CAD build for the part. Positions are in the model's coordinates, mm. A direction names the side the tool comes from. Coordinates: 2 decimals unless noted, no trailing zeros. Loops run counter-clockwise (first coordinate to the right, second up) from the corner with the lowest first, then second, coordinate; pieces in that order, holes last. Notation, with made-up numbers: (17.25, -17.5) -> (37.25, -17.5) arc R25 cw to (37.25, 21.5) -> close; hole circle Ø5 at (-27, 44). An arc over 180 degrees is marked (long way). Return JSON: item names as keys, results as strings. Group by question number.
(1) Probe L1, parallel to Z at x = 0, y = -8; L2, parallel to Y at x = -3.5, z = 11; L3, parallel to X at y = -13.75, z = 10. List the from-to ranges inside material, lowest first.
(2) Mould opens along X. For faces 1 (the face through (15.273, -7.395, -7.126)), 2 (the face through (-15.349, -7.395, -7.108)), 3 (the face through (2.69, -14.88, -5.18)) say: pulls with the +X half, pulls with the -X half, needs draft (parallel to the pull), parting line crosses it, or undercut.
(3) Tool access for faces 4 (the face through (-3, -13, 0)), 5 (the face through (2.057, -7.395, 16.727)), 6 (the face through (-12.34, -7.4, -8.94)), 7 (the face through (-4.731, -7.395, -14.487)): list every direction of +Z, -Z, +X, -X, +Y, -Y with a clear straight run to the whole face (end or side of a thin tool).
(4) Flat gauge pins, fed straight in: pin 1 Ø2 at (x, z) = (-5, 14.5) entering from +Y; pin 2 Ø1 at (x, y) = (-10, -3) entering from +Z; pin 3 Ø4 at (y, z) = (-7, 1.5) entering from -X; pin 4 Ø2 at (x, z) = (-3, -9.5) entering from -Y. Where does each tip first touch, or does it go through?
(5) Saw through at A-A on x = 12.5. Write the cut outline in (y, z).
```python
from build123d import *

# Parameters (mm, degrees)
F1_DEPTH = 15
F2_SIZE  = 0.5
F3_SIZE  = 4
F4_R     = 2
F5_DEPTH = 25.4
F6_R     = 3
F7_DEPTH = 5
F8_R     = 14.605
F8_R_2   = 3.175
F9_DEPTH = 2.54


# Not quite as in the source:
# - a fillet or chamfer that OpenCascade refuses, or shapes differently, is made with other operations: its cross-section is extruded or revolved along the edge and cut away or added


with BuildPart() as f1:
    # F0 (on Front) → F1 (new body)
    with BuildSketch(Plane.XZ):
        with BuildLine():
            Line((0, -20.1), (3.1676147888, -14.9071733253))
            ThreePointArc((3.1676147888, -14.9071733253), (0, -15.24), (-3.1676147888, -14.9071733253))
            Line((-3.1676147888, -14.9071733253), (0, -20.1))
        make_face()
        with BuildLine():
            ThreePointArc((-3.1676147888, 14.9071733253), (0, 15.24), (3.1676147888, 14.9071733253))
            Line((3.1676147888, 14.9071733253), (0, 20.1))
            Line((0, 20.1), (-3.1676147888, 14.9071733253))
        make_face()
        with BuildLine():
            ThreePointArc((-11.3248708297, 10.1982793004), (-8.9578472449, 12.3294189943), (-6.1995624382, 13.922033816))
            Line((-6.1995624382, 13.922033816), (-11.8144835711, 16.2612415869))
            Line((-11.8144835711, 16.2612415869), (-11.3248708297, 10.1982793004))
        make_face()
        with BuildLine():
            ThreePointArc((-15.1564111319, 1.5939892096), (-14.4941013083, 4.7094189943), (-13.1987175292, 7.6191505816))
            Line((-13.1987175292, 7.6191505816), (-19.1162359775, 6.2112415869))
            Line((-19.1162359775, 6.2112415869), (-15.1564111319, 1.5939892096))
        make_face()
        with BuildLine():
            Line((-19.1162359775, -6.2112415869), (-13.1987175292, -7.6191505816))
            ThreePointArc((-13.1987175292, -7.6191505816), (-14.4941013083, -4.7094189943), (-15.1564111319, -1.5939892096))
            Line((-15.1564111319, -1.5939892096), (-19.1162359775, -6.2112415869))
        make_face()
        with BuildLine():
            Line((-11.8144835711, -16.2612415869), (-6.1995624382, -13.922033816))
            ThreePointArc((-6.1995624382, -13.922033816), (-8.9578472449, -12.3294189943), (-11.3248708297, -10.1982793004))
            Line((-11.3248708297, -10.1982793004), (-11.8144835711, -16.2612415869))
        make_face()
        with BuildLine():
            ThreePointArc((15.1564111319, -1.5939892096), (15.2190884361, -0.7980897035), (15.24, 0))
            ThreePointArc((15.24, 0), (15.2190884361, 0.7980897035), (15.1564111319, 1.5939892096))
            ThreePointArc((15.1564111319, 1.5939892096), (14.4941013083, 4.7094189943), (13.1987175292, 7.6191505816))
            ThreePointArc((13.1987175292, 7.6191505816), (12.3294189943, 8.9578472449), (11.3248708297, 10.1982793004))
            ThreePointArc((11.3248708297, 10.1982793004), (8.9578472449, 12.3294189943), (6.1995624382, 13.922033816))
            ThreePointArc((6.1995624382, 13.922033816), (4.7094189943, 14.4941013083), (3.1676147888, 14.9071733253))
            ThreePointArc((3.1676147888, 14.9071733253), (0, 15.24), (-3.1676147888, 14.9071733253))
            ThreePointArc((-3.1676147888, 14.9071733253), (-4.7094189943, 14.4941013083), (-6.1995624382, 13.922033816))
            ThreePointArc((-6.1995624382, 13.922033816), (-8.9578472449, 12.3294189943), (-11.3248708297, 10.1982793004))
            ThreePointArc((-11.3248708297, 10.1982793004), (-12.3294189943, 8.9578472449), (-13.1987175292, 7.6191505816))
            ThreePointArc((-13.1987175292, 7.6191505816), (-14.4941013083, 4.7094189943), (-15.1564111319, 1.5939892096))
            ThreePointArc((-15.1564111319, 1.5939892096), (-15.24, 0), (-15.1564111319, -1.5939892096))
            ThreePointArc((-15.1564111319, -1.5939892096), (-14.4941013083, -4.7094189943), (-13.1987175292, -7.6191505816))
            ThreePointArc((-13.1987175292, -7.6191505816), (-12.3294189943, -8.9578472449), (-11.3248708297, -10.1982793004))
            ThreePointArc((-11.3248708297, -10.1982793004), (-8.9578472449, -12.3294189943), (-6.1995624382, -13.922033816))
            ThreePointArc((-6.1995624382, -13.922033816), (-4.7094189943, -14.4941013083), (-3.1676147888, -14.9071733253))
            ThreePointArc((-3.1676147888, -14.9071733253), (0, -15.24), (3.1676147888, -14.9071733253))
            ThreePointArc((3.1676147888, -14.9071733253), (4.7094189943, -14.4941013083), (6.1995624382, -13.922033816))
            ThreePointArc((6.1995624382, -13.922033816), (8.9578472449, -12.3294189943), (11.3248708297, -10.1982793004))
            ThreePointArc((11.3248708297, -10.1982793004), (12.3294189943, -8.9578472449), (13.1987175292, -7.6191505816))
            ThreePointArc((13.1987175292, -7.6191505816), (14.4941013083, -4.7094189943), (15.1564111319, -1.5939892096))
        make_face()
        with BuildLine():
            ThreePointArc((6.1995624382, 13.922033816), (8.9578472449, 12.3294189943), (11.3248708297, 10.1982793004))
            Line((11.3248708297, 10.1982793004), (11.8144835711, 16.2612415869))
            Line((11.8144835711, 16.2612415869), (6.1995624382, 13.922033816))
        make_face()
        with BuildLine():
            ThreePointArc((13.1987175292, 7.6191505816), (14.4941013083, 4.7094189943), (15.1564111319, 1.5939892096))
            Line((15.1564111319, 1.5939892096), (19.1162359775, 6.2112415869))
            Line((19.1162359775, 6.2112415869), (13.1987175292, 7.6191505816))
        make_face()
        with BuildLine():
            Line((19.1162359775, -6.2112415869), (15.1564111319, -1.5939892096))
            ThreePointArc((15.1564111319, -1.5939892096), (14.4941013083, -4.7094189943), (13.1987175292, -7.6191505816))
            Line((13.1987175292, -7.6191505816), (19.1162359775, -6.2112415869))
        make_face()
        with BuildLine():
            Line((11.8144835711, -16.2612415869), (11.3248708297, -10.1982793004))
            ThreePointArc((11.3248708297, -10.1982793004), (8.9578472449, -12.3294189943), (6.1995624382, -13.922033816))
            Line((6.1995624382, -13.922033816), (11.8144835711, -16.2612415869))
        make_face()
    extrude(amount=F1_DEPTH)

    # F2
    f2_edges = [f1.edges().sort_by_distance(p)[0] for p in [
        (0, -7.5, -20.1),
        (0, -7.5, 20.1),
        (-11.814484, -7.5, -16.261242),
        (-19.116236, -7.5, -6.211242),
        (-19.116236, -7.5, 6.211242),
        (-11.814484, -7.5, 16.261242),
        (11.814484, -7.5, 16.261242),
        (19.116236, -7.5, 6.211242),
        (19.116236, -7.5, -6.211242),
        (11.814484, -7.5, -16.261242),
    ]]
    chamfer(f2_edges, length=F2_SIZE)

    # F3
    f3_edges = [f1.edges().sort_by_distance(p)[0] for p in [
        (-11.563586, -15, 15.915911),
        (-11.563586, 0, 15.915911),
        (0, 0, 19.673148),
        (0, -15, 19.673148),
        (0, -15, -19.673148),
        (-11.563586, -15, -15.915911),
        (-18.710275, -15, -6.079337),
        (-18.710275, -15, 6.079337),
        (-18.710275, 0, 6.079337),
        (-18.710275, 0, -6.079337),
        (-11.563586, 0, -15.915911),
        (0, 0, -19.673148),
        (11.563586, -15, 15.915911),
        (18.710275, -15, 6.079337),
        (18.710275, -15, -6.079337),
        (11.563586, -15, -15.915911),
        (11.563586, 0, 15.915911),
        (18.710275, 0, 6.079337),
        (18.710275, 0, -6.079337),
        (11.563586, 0, -15.915911),
    ]]
    chamfer(f3_edges, length=F3_SIZE)

    # F4 (on face) → F5 (cut)
    with BuildSketch(Plane.XZ.offset(15)):
        Circle(F4_R)
    extrude(amount=-F5_DEPTH, mode=Mode.SUBTRACT)

    # F6 (on face) → F7 (cut)
    with BuildSketch(Plane.XZ.offset(15)):
        Circle(F6_R)
    extrude(amount=-F7_DEPTH, mode=Mode.SUBTRACT)

    # F8 (on face) → F9 (cut)
    with BuildSketch(Plane.XZ.offset(15)):
        Circle(F8_R)
        Circle(F8_R_2, mode=Mode.SUBTRACT)
    extrude(amount=-F9_DEPTH, mode=Mode.SUBTRACT)

    # F10: chamfer of 5.08 on 1 edges, made by hand


with BuildPart() as f10_tool2:
    # F10_s3 → F10_t4 (revolve)
    with BuildSketch(Plane.XY):
        Polygon((8.255, -12.46), (3.175, -17.54), (3.175, -12.46), align=None)
    revolve(axis=Axis((0, -12.46, 0), (0, -1, 0)))

    split(bisect_by=Plane.XZ.offset(15), keep=Keep.BOTTOM)


with BuildPart() as f1_1:
    add(f1.part)

    # F10_t1: union F10_tool2
    add(f10_tool2.part)


solid = f1_1.part
```
Geometry results:
{
 "1": {"L1": "-19.67 to -2, 2 to 19.67", "L2": "-12.46 to 0", "L3": "-11.5 to -10.64, 10.64 to 11.5"},
 "2": {"face 1": "pulls with the +X half", "face 2": "pulls with the -X half", "face 3": "undercut"},
 "3": {"face 4": "-Y", "face 5": "+Z, +Y, -Y", "face 6": "-X, +Y, -Y", "face 7": "-Z, +Y, -Y"},
 "4": {"pin 1": "y = 0", "pin 2": "z = 15.7", "pin 3": "x = -16.79", "pin 4": "y = -12.46"},
 "5": {"outline": "(-15, -8.72) -> (0, -8.72) -> (0, 8.72) -> (-15, 8.72) -> (-15, 7.55) -> (-12.46, 7.55) -> (-12.46, -7.55) -> (-15, -7.55) -> close"}
}
